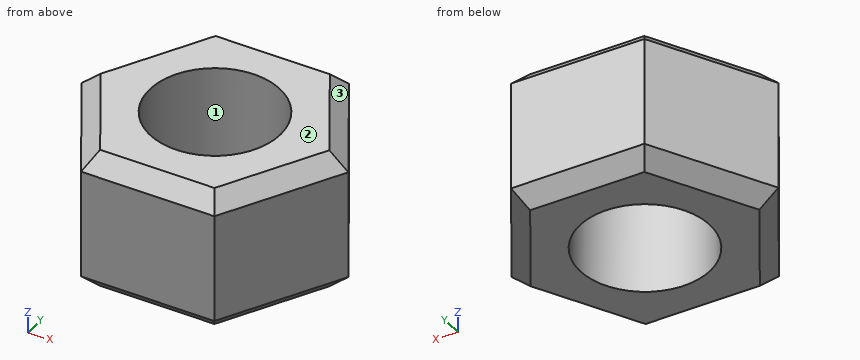
```python
from build123d import *

# Parameters (mm, degrees)
F0_R     = 4
F1_DEPTH = 8.7
F2_SIZE  = 1


with BuildPart() as f1:
    # F0 (on Top) → F1 (new body)
    with BuildSketch(Plane.XY):
        Polygon((4.057701, -6.990594), (8.082882, 0.018775), (4.025181, 7.009369), (-4.057701, 6.990594), (-8.082882, -0.018775), (-4.025181, -7.009369), align=None)
        Circle(F0_R, mode=Mode.SUBTRACT)
    extrude(amount=F1_DEPTH)

    # F2
    f2_edges = [f1.edges().sort_by_distance(p)[0] for p in [
        (-6.070291, 3.485909, 8.7),
        (-6.054032, -3.514072, 8.7),
        (0.01626, -6.999981, 8.7),
        (6.070291, -3.485909, 8.7),
        (6.054032, 3.514072, 8.7),
        (-0.01626, 6.999981, 8.7),
        (-6.070291, 3.485909, 0),
        (-0.01626, 6.999981, 0),
        (-6.054032, -3.514072, 0),
        (0.01626, -6.999981, 0),
        (6.070291, -3.485909, 0),
        (6.054032, 3.514072, 0),
    ]]
    chamfer(f2_edges, length=F2_SIZE)


solid = f1.part
```
Can you work these out from the model? Positions are in its coordinate system, mm. Face numbers are marked on the shaded views. Coordinates: 2 decimals unless noted, no trailing zeros. Loops run counter-clockwise (first coordinate to the right, second up) from the corner with the lowest first, then second, coordinate; pieces in that order, holes last.
1) Thinking about a two-plate mould opening in X: for the marked faces 1, 2 and 3, which applies, pulls with the +X half, pulls with the -X half, needs draft (parallel to the pull), parting line crosses it, or undercut?
2) I need wall thicknesses on probe 1 along X at (y, z) = (-2, 2.5); probe 2 along X at (y, z) = (1.75, 3); probe 3 along Y at (x, z) = (0, 4.75). Which ranges of each line are inside material? Lowest first, please.
3) For pin 1 (2 mm diameter, centred on y = 2, z = 7.5, fed in from -X); pin 2 (2 mm diameter, centred on y = -3, z = 4, fed in from -X), each with a flat end and sliding along its axis, tell me the tip position at first contact or that it passes through.
4) Imagine slicing it at C-C on y = -3.75. List the corners of the cut face in (x, z) for me.
5) Imagine slicing it at A-A on z = 4.25. List the corners of the cut face in (x, y) for me.
6) Imagine slicing it at D-D on y = -5.75. List the corners of the cut face in (x, z) for me, plus the area to 3 significant figures.
7) Imagine slicing it at B-B on x = 0. List the corners of the cut face in (y, z) for me.
Completed:
1. face 1: undercut
1. face 2: needs draft
1. face 3: pulls with the +X half
2. probe 1: x = -6.93 to -3.46, 3.46 to 6.92
2. probe 2: x = -7.07 to -3.6, 3.6 to 7.08
2. probe 3: y = -7 to -4, 4 to 7
3. pin 1: stops at x = -7.5
3. pin 2: stops at x = -6.93
4. outline: (-5.92, 1) - (-4.76, 0) - (-1.39, 0) - (-1.39, 8.7) - (-4.76, 8.7) - (-5.92, 7.7) - close; (1.39, 0) - (4.77, 0) - (5.92, 1) - (5.92, 7.7) - (4.77, 8.7) - (1.39, 8.7) - close
5. outline: (-8.08, -0.02) - (-4.03, -7.01) - (4.06, -6.99) - (8.08, 0.02) - (4.03, 7.01) - (-4.06, 6.99) - close; hole circle Ø8 at (0, 0)
6. outline: (-4.76, 1) - (-3.6, 0) - (3.62, 0) - (4.77, 1) - (4.77, 7.7) - (3.62, 8.7) - (-3.6, 8.7) - (-4.76, 7.7) - close
6. area: 80.6 mm2
7. outline: (-7, 1) - (-6, 0) - (-4, 0) - (-4, 8.7) - (-6, 8.7) - (-7, 7.7) - close; (4, 0) - (6, 0) - (7, 1) - (7, 7.7) - (6, 8.7) - (4, 8.7) - close
